```python
from build123d import *

# Parameters (mm, degrees)
SKETCH_1_W      = 18
SKETCH_1_H      = 12
EXTRUDE_1_DEPTH = 10
EXTRUDE_2_DEPTH = 15
SKETCH_3_R      = 2
EXTRUDE_3_DEPTH = 0.4
EXTRUDE_5_DEPTH = 7.6
SKETCH_5_W      = 12
SKETCH_5_H      = 18.5
EXTRUDE_6_DEPTH = 6.5


with BuildPart() as part:
    # 草图1 → 凸台-拉伸1 (new body)
    with BuildSketch(Plane(origin=(0, 0, 0), x_dir=(1, 0, 0), z_dir=(0, 1, 0))):
        with Locations((9, 6)):
            Rectangle(SKETCH_1_W, SKETCH_1_H)
    extrude(amount=EXTRUDE_1_DEPTH)

    # 草图2 → 凸台-拉伸2 (add)
    with BuildSketch(Plane(origin=(18, 0, 0), x_dir=(0, 0, -1), z_dir=(1, 0, 0))):
        with BuildLine():
            Line((2.68337521, 10), (9.31662479, 10))
            ThreePointArc((9.31662479, 10), (12, 5), (9.31662479, 0))
            Line((9.31662479, 0), (2.68337521, 0))
            ThreePointArc((2.68337521, 0), (0, 5), (2.68337521, 10))
        make_face()
    extrude(amount=EXTRUDE_2_DEPTH)

    # 草图3 → 凸台-拉伸3 (add)
    with BuildSketch(Plane(origin=(0, 10, 0), x_dir=(1, 0, 0), z_dir=(0, 1, 0))):
        with Locations(Location((3.96, 6, 0), (0, 0, 90))):
            Circle(SKETCH_3_R)
    extrude(amount=EXTRUDE_3_DEPTH)

    # 草图4 → 凸台-拉伸5 (add)
    with BuildSketch(Plane(origin=(0, 10.4, 0), x_dir=(1, 0, 0), z_dir=(0, 1, 0))):
        with BuildLine():
            Line((4.96, 4.881966011), (4.96, 7.118033989))
            ThreePointArc((4.96, 7.118033989), (2.46, 6), (4.96, 4.881966011))
        make_face()
    extrude(amount=EXTRUDE_5_DEPTH)

    # 草图5 → 凸台-拉伸6 (add)
    with BuildSketch(Plane(origin=(33, 0, 0), x_dir=(0, 0, -1), z_dir=(1, 0, 0))):
        with Locations((6, 0.75)):
            Rectangle(SKETCH_5_W, SKETCH_5_H)
    extrude(amount=EXTRUDE_6_DEPTH)


solid = part.part
```
Here's how the part is built. I have some questions about the finished solid (model axes, mm). A direction names the side the tool comes from. Give positions to 0.01 mm unless a question says otherwise; leave off trailing zeros. Write each loop counter-clockwise with the first axis right and the second up, starting at its lowest first coordinate (ties: lowest second). Pieces come first, ordered by that corner, then holes. Notation, with made-up numbers: (30, 22) -> (60, 22) arc R10 cw to (60, 27) -> close; hole circle Ø6 at (44, 16). An arc over 180 degrees is marked (long way). Use one line per item in the form item = value.
1) Suppose I cut it at C-C (y = 2.75). Please give me the cut outline in (x, z).
Verdict:
outline = (0, -12) -> (18, -12) -> (18, -11.56) -> (33, -11.56) -> (33, -12) -> (39.5, -12) -> (39.5, 0) -> (33, 0) -> (33, -0.44) -> (18, -0.44) -> (18, 0) -> (0, 0) -> close
2) I'm going to push flat-ended pins straight in: pin 1 (3 mm diameter, centred on x = 12, z = -10, fed in from -Y); pin 2 (1.1 mm diameter, centred on y = 13, z = -6, fed in from +X); pin 3 (2 mm diameter, centred on x = 24, z = -2, fed in from +Y). Where does each tip first touch, or does it pass through?
Verdict:
pin_1 = 0
pin_2 = 4.96
pin_3 = 10
3) Suppose I cut it at D-D (z = -8.75). Please give me the cut outline in (x, y).
Verdict:
outline = (0, 0) -> (33, 0) -> (33, -8.5) -> (39.5, -8.5) -> (39.5, 10) -> (0, 10) -> close
4) Suppose I cut it at B-B (z = -6). Please give me the cut outline in (x, y).
Verdict:
outline = (0, 0) -> (33, 0) -> (33, -8.5) -> (39.5, -8.5) -> (39.5, 10) -> (5.96, 10) -> (5.96, 10.4) -> (4.96, 10.4) -> (4.96, 18) -> (2.46, 18) -> (2.46, 10.4) -> (1.96, 10.4) -> (1.96, 10) -> (0, 10) -> close
5) Suppose I cut it at A-A (x = 3.96). Please give me the cut outline in (y, z), and give its area (3 significant figures).
Verdict:
outline = (0, -12) -> (10, -12) -> (10, -8) -> (10.4, -8) -> (10.4, -7.5) -> (18, -7.5) -> (18, -4.5) -> (10.4, -4.5) -> (10.4, -4) -> (10, -4) -> (10, 0) -> (0, 0) -> close
area = 144 mm2
6) If I drill on L1, parallel to Y at x = 11, z = -2; L2, parallel to X at y = -4.5, z = -0.75; L3, parallel to Y at x = 37, z = -5, over which ranges is the centre line in solid material (lowest first)? Write a range as [from, to].
Verdict:
L1 = [0, 10]
L2 = [33, 39.5]
L3 = [-8.5, 10]
7) On a 3-axis mill with a long thin cutter (end or side, diameter ignored), from which of +Z, -Z, +X, -X, +Y, -Y can I reach the whole of each face in a straight line? I mean faces 1 (the face through (33, 9, -11)), 2 (the face through (4.96, 14, -6)), 3 (the face through (18, 9, -1)), 4 (the face through (18, 1, -1)). Say none if no direction works.
Verdict:
face_1 = -Z, +Y
face_2 = +Z, -Z, +X, +Y
face_3 = +Z, +Y
face_4 = +Z, -Y
